from build123d import *

# Parameters (mm, degrees)
EXTRUDE_1_DEPTH          = 41.5
EXTRUDE_2_DEPTH          = 41.5
CUT_EXTRUDE_1_DEPTH      = 9
CUT_EXTRUDE_1_DEPTH_BACK = 9
SKETCH_5_W               = 311.655321532
SKETCH_5_H               = 249.673450863


with BuildPart() as part:
    # Sketch 1 → Extrude 1 (new body)
    with BuildSketch(Plane(origin=(0, -8, 0), x_dir=(1, 0, 0), z_dir=(0, 1, 0))):
        Polygon((-93.3, -6), (-93.3, -9), (-25, -9), (-14, -6), (8, -6), (8, -3), (-14.401754251, -3), (-25.401754251, -6), align=None)
    extrude(amount=EXTRUDE_1_DEPTH)

    # Sketch 2 → Revolve 1 (revolve)
    with BuildSketch(Plane(origin=(0, 0, 0), x_dir=(0, 0, -1), z_dir=(1, 0, 0)), mode=Mode.PRIVATE) as revolve_1_sk:
        with BuildLine():
            Line((-6, 4.82182538), (-6, 4))
            Line((-6, 4), (6, 4))
            Line((6, 4), (6, 4.5))
            Line((6, 4.5), (7, 4.5))
            Line((7, 4.5), (7, 0))
            Line((7, 0), (-7.5, 0))
            ThreePointArc((-7.5, 0), (-7.11634154, 2.524876235), (-6, 4.82182538))
        make_face()
    revolve(revolve_1_sk.sketch.rotate(Axis((0, 0, -7), (0, 0, 1)), 180), axis=Axis((0, 0, -7), (0, 0, 1)))

    # Sketch 3 → Revolve 2 (revolve)
    with BuildSketch(Plane(origin=(0, 0, 0), x_dir=(0, 0, -1), z_dir=(1, 0, 0)), mode=Mode.PRIVATE) as revolve_2_sk:
        with BuildLine():
            Line((-6, 29.82182538), (-6, 29))
            Line((-6, 29), (6, 29))
            Line((6, 29), (6, 29.5))
            Line((6, 29.5), (7, 29.5))
            Line((7, 29.5), (7, 25))
            Line((7, 25), (-7.5, 25))
            ThreePointArc((-7.5, 25), (-7.11634154, 27.524876235), (-6, 29.82182538))
        make_face()
    revolve(revolve_2_sk.sketch.rotate(Axis((0, 25, -7), (0, 0, 1)), 270), axis=Axis((0, 25, -7), (0, 0, 1)))

    # Sketch 4 → Extrude 2 (add)
    with BuildSketch(Plane(origin=(0, -8, 0), x_dir=(1, 0, 0), z_dir=(0, 1, 0))):
        Polygon((-93.3, 6), (-25.401754251, 6), (-14.401754251, 3), (8, 3), (8, 6), (-14, 6), (-25, 9), (-93.3, 9), align=None)
    extrude(amount=EXTRUDE_2_DEPTH)

    # Sketch 5 → Cut-Extrude 1 (cut, two sides: drawn at the far end of the back side and taken through both)
    with BuildSketch(Plane.XY.offset(-CUT_EXTRUDE_1_DEPTH_BACK)):
        with Locations((-43.959476141, 21.043348893)):
            Rectangle(SKETCH_5_W, SKETCH_5_H)
        with BuildLine():
            Line((-91.3, 13.5), (-21, 13.5))
            ThreePointArc((-21, 13.5), (-11.807611845, 9.692388155), (-8, 0.5))
            Line((-8, 0.5), (-8, 0))
            ThreePointArc((-8, 0), (0, -8), (8, 0))
            Line((8, 0), (8, 25.5))
            ThreePointArc((8, 25.5), (5.656854249, 31.156854249), (0, 33.5))
            Line((0, 33.5), (-91.3, 33.5))
            ThreePointArc((-91.3, 33.5), (-92.714213562, 32.914213562), (-93.3, 31.5))
            Line((-93.3, 31.5), (-93.3, 15.5))
            ThreePointArc((-93.3, 15.5), (-92.714213562, 14.085786438), (-91.3, 13.5))
        make_face(mode=Mode.SUBTRACT)
    extrude(amount=CUT_EXTRUDE_1_DEPTH + CUT_EXTRUDE_1_DEPTH_BACK, mode=Mode.SUBTRACT)


solid = part.part
Geometry check sheet. Reference: the model listing, model coordinates, mm. A direction names the side the tool comes from. Coordinates: 2 decimals unless noted, no trailing zeros. Order: outer loops, then holes, each group sorted by start corner. A loop starts at its lowest first (then second) coordinate and runs counter-clockwise, first axis right, second up. Notation, with made-up numbers: (-5, 39) -> (28, 39) arc R11 ccw to (28, 43) -> close; hole circle Ø3 at (-38.75, 16). An arc over 180 degrees is marked (long way). Use a Markdown table: item, result. Add a question column.
1. Cross-section at B-B (x = -46.5). Enter the section's corners in (y, z), and give its area (3 significant figures).
2. Cross-section at A-A (y = 10). Enter the section's corners in (x, z), and give its area (3 significant figures).
3. Mould release check, pull along X, two halves, no side actions. Record for faces 6 (the face through (-19.98, 22.45, -4.52)), 7 (the face through (-3, 17, 6)), 8 (the face through (-60, 23, -6)): pulls with the +X half, pulls with the -X half, needs draft (parallel to the pull), parting line crosses it, or undercut.
4. Cross-section at C-C (z = 1.25). Enter the section's corners in (x, y).
5. Material ranges on L1, parallel to Z at x = -50.5, y = 28.5; L2, parallel to Y at x = -16, z = 4.5; L3, parallel to Z at x = -3.5, y = 22, recorded low to high.
6. Set-up check for faces 1 (the face through (-3.905, 0.867, -0.042)), 2 (the face through (-19.42, 22.32, -7.48)), 3 (the face through (-19.58, 22.32, 7.52)), 4 (the face through (-0.59, 29.46, -6.51)), 5 (the face through (-59, 23, 6)): record each of +Z, -Z, +X, -X, +Y, -Y from which the full face is reachable in a straight line by a thin tool's end or side.
7. Go/stop test with flat-tipped pins: pin 1 Ø11 at (x, y) = (2, 21.5) entering from -Z; pin 2 Ø8 at (y, z) = (3.5, 0) entering from -X; pin 3 Ø11 at (x, y) = (2, 20) entering from +Z; pin 4 Ø10 at (y, z) = (11.5, 4) entering from -X. Record where each tip stops, or that it passes through.
Filled sheet:
| question | item | result |
|---|---|---|
| 1 | outline | (13.5, -9) -> (33.5, -9) -> (33.5, -6) -> (13.5, -6) -> close; (13.5, 6) -> (33.5, 6) -> (33.5, 9) -> (13.5, 9) -> close |
| 1 | area | 120 mm2 |
| 2 | outline | (-12.13, -6) -> (8, -6) -> (8, -3) -> (-12.13, -3) -> close; (-12.13, 3) -> (8, 3) -> (8, 6) -> (-12.13, 6) -> close |
| 2 | area | 121 mm2 |
| 3 | face 6 | pulls with the -X half |
| 3 | face 7 | undercut |
| 3 | face 8 | needs draft |
| 4 | outline | circle Ø8 at (0, 0); circle Ø8 at (0, 25) |
| 5 | L1 | -9 to -6, 6 to 9 |
| 5 | L2 | 12.5 to 33.5 |
| 5 | L3 | -6 to -3, 3 to 6.14 |
| 6 | face 1 | none |
| 6 | face 2 | -Z, +Y, -Y |
| 6 | face 3 | +Z, +Y, -Y |
| 6 | face 4 | -Z |
| 6 | face 5 | -X, +Y, -Y |
| 7 | pin 1 | z = -7 |
| 7 | pin 2 | x = -9.29 |
| 7 | pin 3 | z = 7.5 |
| 7 | pin 4 | x = -93.3 |
